Autodesk Inventor part; units mm, degrees
ref_plane "YZ Plane" through (0, 0, 0) normal (1, 0, 0) x (0, 1, 0)
ref_plane "XZ Plane" through (0, 0, 0) normal (0, 1, 0) x (-1, 0, 0)
ref_plane "XY Plane" through (0, 0, 0) normal (0, 0, 1) x (1, 0, 0)
sketch "Esquisse1" plane through (0, 0, 0) normal (0, 0, 1) x (1, 0, 0)
  circle A0 centre (0, 0) radius 155
  circle A1 centre (0, 0) radius 275
  line L0 (-275, 0) -> (275, 0)
  line L1 (-155, 0) -> (155, 0)
  circle A2 centre (-175, 5) radius 1.5
  circle A3 centre (175, 5) radius 1.5
  point P0 (-86.6478, -260.9927)
  point P1 (93.3373, -258.6758)
  dimension "d0" = 310
  dimension "d1" = 550
  dimension "d2" = 180
  dimension "d5" = 179.9851
  dimension "d6" = 5
  dimension "d7" = -175
  dimension "d8" = 3
  dimension "d19" = 5
  dimension "d20" = 175
  dimension "d21" = 3
extrude "Extrusion1" add sketch "Esquisse1" along normal mid plane 10 contours L0 A0 | A0 L0 A1 | A2 | A3 picked at (36.5339, 36.5339) picked at (197.6975, 36.6731)
sketch "Esquisse2" plane through (0, 0, 5) normal (0, 0, 1) x (-1, 0, 0)
  arc A0 (-275, 0) -> (275, 0) centre (0, 0) ccw
  line L0 (-275, 0) -> (275, 0)
sketch "Esquisse3" plane through (0, 0, -5) normal (0, 0, -1) x (-1, 0, 0)
  circle A0 centre (175, 5) radius 1.5
  line L0 (275, 0) -> (-275, 0)
  point P0 (0, 0)
  point P1 (155, 0)
  dimension "d9" = 175
  dimension "d10" = 5
  dimension "d11" = 3
extrude "Extrusion2" cut sketch "Esquisse3" against normal blind 10
sketch "Esquisse4" plane through (0, 0, -5) normal (0, 0, -1) x (-1, 0, 0)
  circle A0 centre (255, 5) radius 1.5
  line L0 (-275, 0) -> (275, 0)
  point P0 (0, 0)
  point P1 (155, 0)
  dimension "d14" = 5
  dimension "d15" = 255
  dimension "d16" = 3
extrude "Extrusion3" cut sketch "Esquisse4" against normal blind 10
sketch "Esquisse5" plane through (0, 0, 5) normal (0, 0, 1) x (1, 0, 0)
  circle A0 centre (175, 5) radius 1.5
  line L0 (-275, 0) -> (275, 0)
  circle A1 centre (255, 5) radius 1.5
  point P0 (0, 0)
  point P1 (0, 0)
  point P2 (0, 0)
  dimension "d22" = 5
  dimension "d23" = 3
  dimension "d24" = 175
  dimension "d25" = 255
  dimension "d26" = 3
extrude "Extrusion4" cut sketch "Esquisse5" against normal blind 10 contours A0
sketch "Esquisse6" plane through (0, 0, 5) normal (0, 0, 1) x (1, 0, 0)
  circle A0 centre (255, 5) radius 1.5
  line L0 (-275, 0) -> (275, 0)
  point P0 (0, 0)
  point P1 (0, 0)
  dimension "d31" = 5
  dimension "d32" = 255
  dimension "d33" = 3
extrude "Extrusion6" cut sketch "Esquisse6" against normal blind 10
sketch "Esquisse7" plane through (0, 0, 5) normal (0, 0, 1) x (1, 0, 0)
  circle A0 centre (163.155, 63.48) radius 1.5
  line L0 (-275, 0) -> (275, 0)
  circle A1 centre (237.69, 92.48) radius 1.5
  point P0 (0, 0)
  point P1 (0, 0)
  point P2 (0, 0)
  dimension "d37" = 3
  dimension "d38" = 63.48
  dimension "d39" = 163.155
  dimension "d40" = 92.48
  dimension "d41" = 237.69
  dimension "d42" = 3
extrude "Extrusion7" cut sketch "Esquisse7" against normal blind 10
sketch "Esquisse8" plane through (0, 0, 5) normal (0, 0, 1) x (1, 0, 0)
  circle A0 centre (132.327, 114.625) radius 1.5
  line L0 (-275, 0) -> (275, 0)
  circle A1 centre (192.779, 166.991) radius 1.5
  circle A2 centre (86.1, 152.433) radius 1.5
  circle A3 centre (125.43, 222.071) radius 1.5
  circle A4 centre (29.85, 172.5) radius 1.5
  circle A5 centre (43.499, 251.312) radius 1.5
  line L1 (0, 0) -> (0, 275.6506)
  dimension "d45" = 114.625
  dimension "d46" = 132.327
  dimension "d47" = 3
  dimension "d48" = 166.991
  dimension "d49" = 192.779
  dimension "d50" = 3
  dimension "d51" = 152.433
  dimension "d52" = 86.1
  dimension "d53" = 3
  dimension "d54" = 222.071
  dimension "d55" = 125.43
  dimension "d56" = 3
  dimension "d57" = 172.5
  dimension "d58" = 29.85
  dimension "d59" = 3
  dimension "d60" = 251.312
  dimension "d61" = 43.499
  dimension "d62" = 3
extrude "Extrusion8" cut sketch "Esquisse8" against normal blind 10
sketch "Esquisse9" plane through (0, 0, 5) normal (0, 0, 1) x (1, 0, 0)
  circle A0 centre (-163.155, 63.48) radius 1.5
  circle A1 centre (-237.69, 92.48) radius 1.5
  circle A2 centre (-132.327, 114.625) radius 1.5
  circle A3 centre (-192.779, 166.991) radius 1.5
  circle A4 centre (-86.1, 152.433) radius 1.5
  circle A5 centre (-125.43, 222.071) radius 1.5
  circle A6 centre (-29.85, 172.5) radius 1.5
  circle A7 centre (-43.499, 251.312) radius 1.5
  line L0 (-275, 0) -> (275, 0)
  point P0 (0, 0)
  point P1 (0, 0)
  point P2 (0, 0)
  point P3 (0, 0)
  point P4 (0, 0)
  point P5 (0, 0)
  point P6 (0, 0)
  point P7 (0, 0)
  point P8 (0, 0)
  dimension "d65" = 63.48
  dimension "d66" = 163.155
  dimension "d67" = 3
  dimension "d68" = 92.48
  dimension "d69" = 237.69
  dimension "d70" = 3
  dimension "d71" = 132.327
  dimension "d72" = 114.625
  dimension "d73" = 3
  dimension "d74" = 166.991
  dimension "d75" = 192.779
  dimension "d76" = 3
  dimension "d77" = 152.433
  dimension "d78" = 86.1
  dimension "d79" = 3
  dimension "d80" = 125.43
  dimension "d81" = 222.071
  dimension "d82" = 3
  dimension "d83" = 29.85
  dimension "d84" = 172.5
  dimension "d85" = 3
  dimension "d86" = 43.499
  dimension "d87" = 251.312
  dimension "d88" = 3
extrude "Extrusion9" cut sketch "Esquisse9" against normal blind 10
sketch "Esquisse11" plane through (0, 0, 5) normal (0, 0, 1) x (1, 0, 0)
  line L0 (275, 0) -> (-275, 0)
  line L1 (-275, 0) -> (275, 0)
  line L2 (275, 0) -> (275, -20)
  line L3 (275, -20) -> (-275, -20)
  line L4 (-275, -20) -> (-275, 0)
  point P0 (0, 0)
  dimension "d91" = 20
extrude "Extrusion10" add sketch "Esquisse11" against normal blind 10
sketch "Esquisse12" plane through (0, 0, 5) normal (0, 0, 1) x (1, 0, 0)
  circle A0 centre (0, 0) radius 6
  dimension "d94" = 12
extrude "Extrusion11" cut sketch "Esquisse12" against normal blind 10
properties part number "plaque dessus"
Geometry check sheet. Reference: the model listing, model coordinates, mm. Round coordinates to 2 decimals unless told otherwise and drop trailing zeros. Write each loop counter-clockwise with the first axis right and the second up, starting at its lowest first coordinate (ties: lowest second). Pieces come first, ordered by that corner, then holes. Notation, with made-up numbers: (-35, 73) - (13, 73) arc R31 ccw to (13, 99) - close; hole circle Ø8 at (28.25, 52.25). An arc over 180 degrees is marked (long way). One line per item, written item: value.
1. Cross-section at C-C on y = 122.5. Record the boundary of the cut face in (x, z), and give its area (3 significant figures).
The answers:
outline: (-246.21, -5) - (246.21, -5) - (246.21, 5) - (-246.21, 5) - close
area: 4,920 mm^2
2. Scan lines: L1, parallel to Y at x = 29.85, z = -0.25; L2, parallel to Y at x = -198.5, z = -2.5; L3, parallel to Y at x = -16, z = 2.25. Record each from-to range of solid material in increasing order.
The answers:
L1: y = -20 to 171, 174 to 273.38
L2: y = -20 to 190.32
L3: y = -20 to 274.53
3. Depth check by flat-ended pin: pin 1 Ø1.8 at (x, y) = (-43.499, 251.312) entering from +Z; pin 2 Ø1 at (y, z) = (16.5, 2) entering from +X; pin 3 Ø1 at (x, z) = (206, -3) entering from +Y; pin 4 Ø1 at (x, z) = (72, 3.5) entering from +Y. Enter the tip coordinate at first touch or a pass-through.
The answers:
pin 1: passes through
pin 2: stops at x = 274.53
pin 3: stops at y = 182.74
pin 4: stops at y = 265.54
4. Cross-section at B-B on y = 193.5. Record the boundary of the cut face in (x, z), and give its area (3 significant figures).
The answers:
outline: (-195.4, -5) - (195.4, -5) - (195.4, 5) - (-195.4, 5) - close
area: 3,910 mm^2
5. Mould release check, pull along Y, two halves, no side actions. Record for faces 1 (the face through (-6.047, 274.934, -0.07)), 2 (the face through (-4, 97, -5)), 3 (the face through (-6, 0, 0)), 4 (the face through (4, -20, 0)): released by +Y, released by -Y, zero draft, split by the parting line, or undercut.
The answers:
face 1: released by +Y
face 2: zero draft
face 3: undercut
face 4: released by -Y
6. Cross-section at A-A on z = 0.5. Give the number of separate pieces and of enclosed holes in the cut face, and give its area (3 significant figures).
The answers:
separate pieces: 1
enclosed holes: 21
area: 130,000 mm^2
